Verification items for this drawing (mm, ordinates from the low corner). Round coordinates to 2 decimals unless told otherwise and drop trailing zeros. Write each loop counter-clockwise with the first axis right and the second up, starting at its lowest first coordinate (ties: lowest second). Pieces come first, ordered by that corner, then holes. Notation, with made-up numbers: (-1, 24.25) -> (54, 24.25) arc R25 ccw to (54, 56.25) -> close; hole circle Ø11 at (18.5, -38). An arc over 180 degrees is marked (long way). Use one line per item in the form item = value. Start each with the question number.
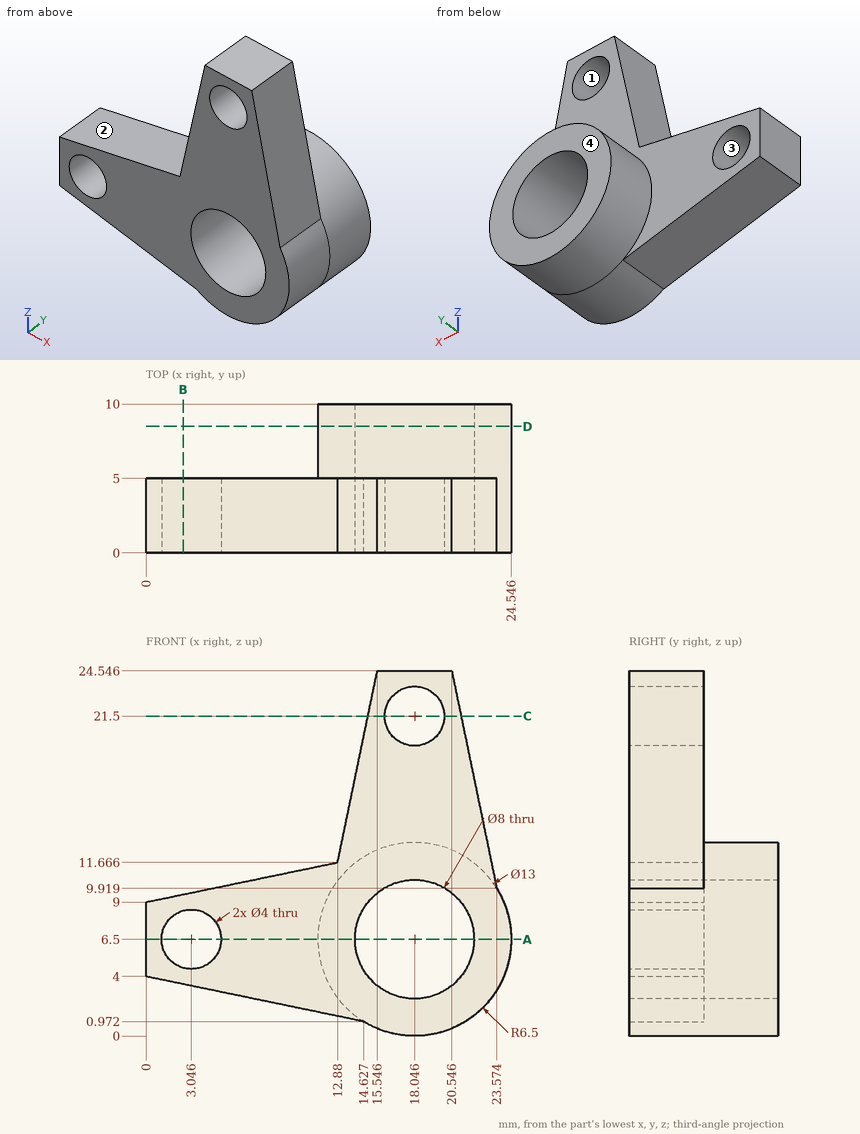
1. Sectioned sample at A-A (z = 6.5). Enter the section's corners in (x, y).
2. Depth check by flat-ended pin: pin 1 (3 mm diameter, centred on y = 5.5, z = 12.5, fed in from +X); pin 2 (1 mm diameter, centred on y = 4.5, z = 12.5, fed in from +X); pin 3 (5 mm diameter, centred on x = 21.5, y = 6, fed in from -Z); pin 4 (10.5 mm diameter, centred on x = 18.05, z = 6.5, fed in from -Y). Enter the tip coordinate at first touch or a pass-through.
3. Sectioned sample at C-C (z = 21.5). Enter the section's corners in (x, y) (1 decimal), and give its area (3 significant figures).
4. Sectioned sample at D-D (y = 8.5). Enter the section's corners in (x, z).
5. Sectioned sample at B-B (x = 2.5). Enter the section's corners in (y, z).
6. Mould release check, pull along Z, two halves, no side actions. Record for the marked faces 1, 2, 3 and 4: +Z half, -Z half, draft (parallel to the pull), parting line (faces both ways), or undercut.
7. Scan lines: probe 1 along X at (y, z) = (5.5, 6.5); probe 2 along Z at (x, y) = (16.75, 1) (1 decimal); probe 3 along Z at (x, y) = (19.5, 2) (1 decimal). Record each from-to range of solid material in increasing order.
Returned:
q1.outline = (0, 0) -> (1.05, 0) -> (1.05, 5) -> (0, 5) -> close; (5.05, 0) -> (14.05, 0) -> (14.05, 10) -> (11.55, 10) -> (11.55, 5) -> (5.05, 5) -> close; (22.05, 0) -> (24.55, 0) -> (24.55, 10) -> (22.05, 10) -> close
q2.pin_1 = 23.33
q2.pin_2 = 23.14
q2.pin_3 = 0.07
q2.pin_4 = 0
q3.outline = (14.9, 0) -> (16, 0) -> (16, 5) -> (14.9, 5) -> close; (20, 0) -> (21.2, 0) -> (21.2, 5) -> (20, 5) -> close
q3.area = 11.3 mm^2
q4.outline = circle Ø13 at (18.05, 6.5); hole circle Ø8 at (18.05, 6.5)
q5.outline = (0, 3.48) -> (5, 3.48) -> (5, 4.58) -> (0, 4.58) -> close; (0, 8.42) -> (5, 8.42) -> (5, 9.52) -> (0, 9.52) -> close
q6.face_1 = undercut
q6.face_2 = +Z half
q6.face_3 = undercut
q6.face_4 = draft
q7.probe_1 = 11.55 to 14.05, 22.05 to 24.55
q7.probe_2 = 0.1 to 2.7, 10.3 to 20, 23 to 24.5
q7.probe_3 = 0.2 to 2.8, 10.2 to 20.1, 22.9 to 24.5
